Geometry check sheet. Reference: the model listing, model coordinates, mm. A direction names the side the tool comes from. Round coordinates to 2 decimals unless told otherwise and drop trailing zeros. Write each loop counter-clockwise with the first axis right and the second up, starting at its lowest first coordinate (ties: lowest second). Pieces come first, ordered by that corner, then holes.
from build123d import *

# Parameters (mm, degrees)
SKETCH1_R           = 11.1
BOSS_EXTRUDE1_DEPTH = 7
SKETCH4_W           = 35
SKETCH4_H           = 20
BOSS_EXTRUDE3_DEPTH = 5
SKETCH5_R           = 2.6
CUT_EXTRUDE1_DEPTH  = 8
BOSS_EXTRUDE4_DEPTH = 2
SKETCH9_W           = 35
SKETCH9_H           = 5
BOSS_EXTRUDE5_DEPTH = 25
SKETCH10_R          = 2.6
CUT_EXTRUDE2_DEPTH  = 25
SKETCH11_W          = 35
SKETCH11_H          = 0.4
CUT_EXTRUDE3_DEPTH  = 4


with BuildPart() as part:
    # Sketch1 → Boss-Extrude1 (new body)
    with BuildSketch(Plane(origin=(0, 0, 0), x_dir=(1, 0, 0), z_dir=(0, 1, 0))):
        with BuildLine():
            Line((-17.5, 0), (-17.5, -15))
            Line((-17.5, -15), (17.5, -15))
            Line((17.5, -15), (17.5, 0))
            ThreePointArc((17.5, 0), (0, 17.5), (-17.5, 0))
        make_face()
        Circle(SKETCH1_R, mode=Mode.SUBTRACT)
    extrude(amount=BOSS_EXTRUDE1_DEPTH)

    # Sketch4 → Boss-Extrude3 (add)
    with BuildSketch(Plane(origin=(0, 0, 0), x_dir=(1, 0, 0), z_dir=(0, 1, 0))):
        with Locations((0, -25)):
            Rectangle(SKETCH4_W, SKETCH4_H)
    extrude(amount=BOSS_EXTRUDE3_DEPTH)

    # Sketch5 → Cut-Extrude1 (cut, through all)
    with BuildSketch(Plane(origin=(0, 7, 0), x_dir=(1, 0, 0), z_dir=(0, 1, 0))):
        with Locations((-11.5, -25)):
            Circle(SKETCH5_R)
        with Locations((11.5, -25)):
            Circle(SKETCH5_R)
    extrude(amount=-CUT_EXTRUDE1_DEPTH, mode=Mode.SUBTRACT)

    # Sketch8 → Boss-Extrude4 (add)
    with BuildSketch(Plane(origin=(0, 7, 0), x_dir=(1, 0, 0), z_dir=(0, 1, 0))):
        with BuildLine():
            Line((-17.5, 0), (-17.5, -15))
            Line((-17.5, -15), (17.5, -15))
            Line((17.5, -15), (17.5, 0))
            ThreePointArc((17.5, 0), (0, 17.5), (-17.5, 0))
        make_face()
    extrude(amount=BOSS_EXTRUDE4_DEPTH)

    # Sketch9 → Boss-Extrude5 (add)
    with BuildSketch(Plane.XZ):
        with Locations((0, 37.5)):
            Rectangle(SKETCH9_W, SKETCH9_H)
    extrude(amount=-BOSS_EXTRUDE5_DEPTH)

    # Sketch10 → Cut-Extrude2 (cut)
    with BuildSketch(Plane(origin=(0, 0, 35), x_dir=(-1, 0, 0), z_dir=(0, 0, -1))):
        with Locations((-11.5, 15)):
            Circle(SKETCH10_R)
        with Locations((11.5, 15)):
            Circle(SKETCH10_R)
    extrude(amount=-CUT_EXTRUDE2_DEPTH, mode=Mode.SUBTRACT)

    # Sketch11 → Cut-Extrude3 (cut)
    with BuildSketch(Plane(origin=(0, 9, 0), x_dir=(1, 0, 0), z_dir=(0, 1, 0))):
        with Locations((0, -14.8)):
            Rectangle(SKETCH11_W, SKETCH11_H)
    extrude(amount=-CUT_EXTRUDE3_DEPTH, mode=Mode.SUBTRACT)


solid = part.part
1. Section check C-C (z = 25). Record the cut outline in (x, y).
2. Section check B-B (y = 15). Record the cut outline in (x, z), plus the area to 3 significant figures.
3. Depth check by flat-ended pin: pin 1 Ø6 at (x, z) = (12, 4) entering from +Y; pin 2 Ø1.5 at (x, y) = (-8, 22.5) entering from -Z. Enter the tip coordinate at first touch or a pass-through.
4. Section check D-D (y = 3.25). Record the cut outline in (x, z).
5. Scan lines: line 1 along X through (y, z) = (3.25, 25); line 2 along Y through (x, z) = (11.5, 36.85); line 3 along Z through (x, y) = (-2, 6.5). Record each from-to range of solid material in increasing order.
6. Section check A-A (x = -10.5). Record the cut outline in (y, z), plus the area to 3 significant figures.
7. Access from +Z, -Z, +X, -X, +Y, -Y to the whole of each face (thin tool, end or side, straight path). Record for faces 1 (the face through (0, 25, 38)), 2 (the face through (-11.838, 2.535, 22.422)), 3 (the face through (0, 7, 0)), 4 (the face through (0, 7, 14.6)), 5 (the face through (0, 9, -2)).
8. Release check for a two-part mould opening along X. For faces 6 (the face through (0, 15, 35)), 7 (the face through (0.385, 4.437, -17.496)), 8 (the face through (5.97, 3.45, -9.36)) record: +X half, -X half, draft (parallel to the pull), parting line (faces both ways), or undercut.
Results below:
1. outline: (-17.5, 0) - (-14.1, 0) - (-14.1, 5) - (-17.5, 5) - close; (-8.9, 0) - (8.9, 0) - (8.9, 5) - (-8.9, 5) - close; (14.1, 0) - (17.5, 0) - (17.5, 5) - (14.1, 5) - close
2. outline: (-17.5, 35) - (-14.1, 35) - (-14.1, 40) - (-17.5, 40) - close; (-8.9, 35) - (8.9, 35) - (8.9, 40) - (-8.9, 40) - close; (14.1, 35) - (17.5, 35) - (17.5, 40) - (14.1, 40) - close
2. area: 123 mm2
3. pin 1: stops at y = 9
3. pin 2: stops at z = 35
4. outline: (-17.5, 0) arc R17.5 ccw to (17.5, 0) - (17.5, 40) - (-17.5, 40) - close; hole circle Ø5.2 at (-11.5, 25); hole circle Ø22.2 at (0, 0); hole circle Ø5.2 at (11.5, 25)
5. line 1: x = -17.5 to -14.1, -8.9 to 8.9, 14.1 to 17.5
5. line 2: y = 0 to 12.4, 17.6 to 25
5. line 3: z = -17.39 to -10.92, 10.92 to 14.6, 35 to 40
6. outline: (0, -14) - (9, -14) - (9, 14.6) - (5, 14.6) - (5, 22.6) - (0, 22.6) - (0, 3.6) - (7, 3.6) - (7, -3.6) - (0, -3.6) - close; (0, 27.4) - (5, 27.4) - (5, 35) - (12.6, 35) - (12.6, 40) - (0, 40) - close; (17.4, 35) - (25, 35) - (25, 40) - (17.4, 40) - close
6. area: 386 mm2
7. face 1: +Z, -Z, +X, -X, +Y
7. face 2: +Y, -Y
7. face 3: -Y
7. face 4: +X, -X, +Y
7. face 5: -Z, +X, -X, +Y
8. face 6: draft
8. face 7: parting line
8. face 8: undercut
